Build history of the part. All positions in model axes, mm. Face numbers are marked on the shaded views. A direction names the side the tool comes from. Round coordinates to 2 decimals unless told otherwise and drop trailing zeros. Order: outer loops, then holes, each group sorted by start corner. A loop starts at its lowest first (then second) coordinate and runs counter-clockwise, first axis right, second up. Notation, with made-up numbers: (61, 56.5) -> (116, 56.5) arc R24 cw to (116, 68.5) -> close; hole circle Ø9 at (85.5, 60.5). An arc over 180 degrees is marked (long way). Answer as a JSON object with one key per item and string values.
from build123d import *

# Parameters (mm, degrees)
F0_W     = 254
F0_H     = 254
F1_DEPTH = 203.2
F2_SIZE2 = 127
F2_SIZE  = 50.8
F3_T     = -2.54


with BuildPart() as f1:
    # F0 (on Front) → F1 (new body)
    with BuildSketch(Plane.XZ):
        with Locations((127, 127)):
            Rectangle(F0_W, F0_H)
    extrude(amount=F1_DEPTH)

    # F2
    f2_edges = [f1.edges().sort_by_distance(p)[0] for p in [
        (127, -203.2, 254),
        (127, 0, 0),
    ]]
    chamfer(f2_edges, length=F2_SIZE, length2=F2_SIZE2)

    # F3
    f3_openings = [f1.faces().sort_by_distance(p)[0] for p in [
        (254, -101.6, 127),
    ]]
    offset(amount=F3_T, openings=f3_openings)


solid = f1.part
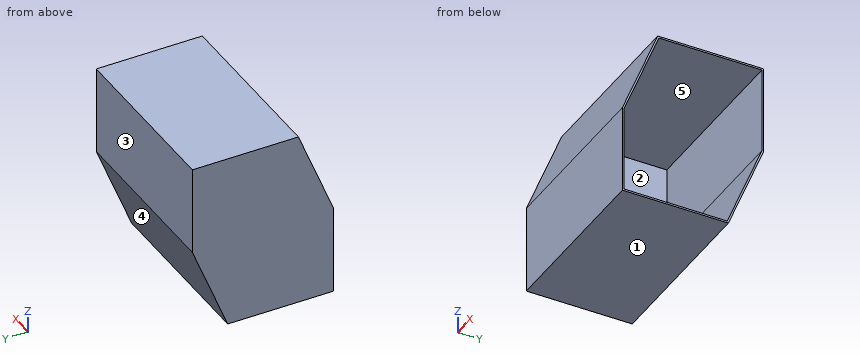
1) Probe L1, parallel to Z at x = 230, y = -100; L2, parallel to X at y = -120, z = 30; L3, parallel to Y at x = 174, z = 112. List the from-to ranges inside material, lowest first. Write a range as from..to.
Checked values:
{"L1": "z = 0..2.54, 251.46..254", "L2": "x = 0..2.54", "L3": "y = -203.2..-200.66, -8.74..-6"}
2) Cut at A-A, the plane y = -107.5. Give the cut face in (x, z), plus the area to 3 significant figures.
Checked values:
{"outline": "(0, 0) -> (254, 0) -> (254, 2.54) -> (2.54, 2.54) -> (2.54, 251.46) -> (254, 251.46) -> (254, 254) -> (0, 254) -> close", "area": "1,920 mm²"}
3) Which spindle directions (+Z, -Z, +X, -X, +Y, -Y) get a long thin tool onto all of the face, cutting with end or side? Do the marked faces 1 and 2. Say none if no direction does.
Checked values:
{"face 1": "-Z, +X, -X, +Y, -Y", "face 2": "+X"}
4) Cut at B-B, the plane x = 130. Give the cut face in (y, z).
Checked values:
{"outline": "(-203.2, 0) -> (-50.8, 0) -> (0, 127) -> (0, 254) -> (-152.4, 254) -> (-203.2, 127) -> close; hole (-200.66, 2.54) -> (-52.52, 2.54) -> (-2.54, 127.49) -> (-2.54, 251.46) -> (-150.68, 251.46) -> (-200.66, 126.51) -> close"}
5) Flat gauge pins, fed straight in: pin 1 Ø12 at (x, z) = (128.5, 34) entering from +Y; pin 2 Ø3 at (x, z) = (34.5, 40) entering from +Y; pin 3 Ø4 at (y, z) = (-45.5, 164) entering from +X. Where does each tip first touch, or does it go through?
Checked values:
{"pin 1": "stops at y = -34.8", "pin 2": "stops at y = -34.2", "pin 3": "stops at x = 2.54"}
6) Cut at C-C, the plane z = 232.5. Give the cut face in (x, y).
Checked values:
{"outline": "(0, -161) -> (254, -161) -> (254, -158.26) -> (2.54, -158.26) -> (2.54, -2.54) -> (254, -2.54) -> (254, 0) -> (0, 0) -> close"}
7) Pull direction Z, two halves, no side cores. Call the marked faces 3, 4 and 5: pulls with the +Z half, pulls with the -Z half, needs draft (parallel to the pull), parting line crosses it, or undercut.
Checked values:
{"face 3": "needs draft", "face 4": "pulls with the -Z half", "face 5": "undercut"}
